```python
from build123d import *

# Parameters (mm, degrees)
SKETCH1_R                      = 3.81
BOSS_EXTRUDE1_DEPTH            = 12.7
CUT_EXTRUDE1_REACH             = 5.81
SKETCH2_R                      = 1.905
CUT_EXTRUDE1_DIRECTION_2_DEPTH = 19.05


with BuildPart() as part:
    # Sketch1 → Boss-Extrude1 (new body)
    with BuildSketch(Plane(origin=(0, 0, 0), x_dir=(1, 0, 0), z_dir=(0, 1, 0))):
        Circle(SKETCH1_R)
    extrude(amount=BOSS_EXTRUDE1_DEPTH)

    # Sketch2 → Cut-Extrude1 (cut, up to next)
    with BuildSketch(Plane.XY, mode=Mode.PRIVATE) as cut_extrude1_sk1:
        with Locations((0, 8.89)):
            Circle(SKETCH2_R)
    cut_extrude1_tool1 = extrude(cut_extrude1_sk1.sketch, amount=-CUT_EXTRUDE1_REACH, mode=Mode.PRIVATE) & part.part
    add(cut_extrude1_tool1.solids().sort_by_distance((0, 8.89, 0))[0], mode=Mode.SUBTRACT)

    # Sketch2 → Cut-Extrude1 direction 2 (cut)
    with BuildSketch(Plane.XY):
        with Locations((0, 8.89)):
            Circle(SKETCH2_R)
    extrude(amount=CUT_EXTRUDE1_DIRECTION_2_DEPTH, mode=Mode.SUBTRACT)


solid = part.part
```
Part model, mm, in its own coordinate system. Give positions to 0.01 mm unless a question says otherwise; leave off trailing zeros. Write each loop counter-clockwise with the first axis right and the second up, starting at its lowest first coordinate (ties: lowest second). Pieces come first, ordered by that corner, then holes. Notation, with made-up numbers: (-4, 64) -> (22, 64) arc R12 cw to (22, 87) -> close; hole circle Ø4 at (31, 29). An arc over 180 degrees is marked (long way). Put each result on its own line as item: value. Start each with the question number.
Item 1: Cut at D-D (y = 3.75). List the corners of the cut face in (x, z), then the cut area to 3 significant figures.
Item 2: Cut at C-C (y = 9.75). List the corners of the cut face in (x, z).
Item 3: Cut at A-A (x = 0). List the corners of the cut face in (y, z) (3 decimals).
Item 4: Pull direction Y, two halves, no side cores. Call faces 1 (the face through (1.817, 9.462, 0.053)), 2 (the face through (0, 0, 0)), 3 (the face through (0, 12.7, 0)): pulls with the +Y half, pulls with the -Y half, needs draft (parallel to the pull), parting line crosses it, or undercut.
Item 5: Wall check: L1, parallel to Y at x = 0, z = -0.25 (3 decimals); L2, parallel to X at y = 8.89, z = 0 (3 decimals); L3, parallel to X at y = 8.25, z = 2. Give the ranges that are in metal, low to high. Write a range as [from, to].
Item 6: Cut at B-B (z = 0). List the corners of the cut face in (x, y) (3 decimals), then the cut area to 3 significant figures.
Item 7: Pin check, flat tips, straight feed: pin 1 Ø3 at (y, z) = (2.5, -2) entering from -X; pin 2 Ø1.5 at (x, y) = (1, 4.5) entering from -Z; pin 3 Ø1 at (x, y) = (1, 7) entering from +Z. Stop position of each tip, or through.
Answer list:
1. outline: circle Ø7.62 at (0, 0)
1. area: 45.6 mm2
2. outline: (-1.7, -3.41) -> (-1.7, 3.41) arc R3.81 ccw to start; (1.7, -3.41) arc R3.81 ccw to (1.7, 3.41) -> close
3. outline: (0, -3.81) -> (6.985, -3.81) -> (6.985, 3.81) -> (0, 3.81) -> close; (10.795, -3.81) -> (12.7, -3.81) -> (12.7, 3.81) -> (10.795, 3.81) -> close
4. face 1: undercut
4. face 2: pulls with the -Y half
4. face 3: pulls with the +Y half
5. L1: y = [0, 6.985], [10.795, 12.7]
5. L2: x = [-3.81, -1.905], [1.905, 3.81]
5. L3: x = [-3.24, -1.79], [1.79, 3.24]
6. outline: (-3.81, 0) -> (3.81, 0) -> (3.81, 12.7) -> (-3.81, 12.7) -> close; hole circle Ø3.81 at (0, 8.89)
6. area: 85.4 mm2
7. pin 1: stops at x = -3.78
7. pin 2: stops at z = -3.8
7. pin 3: stops at z = 3.78
